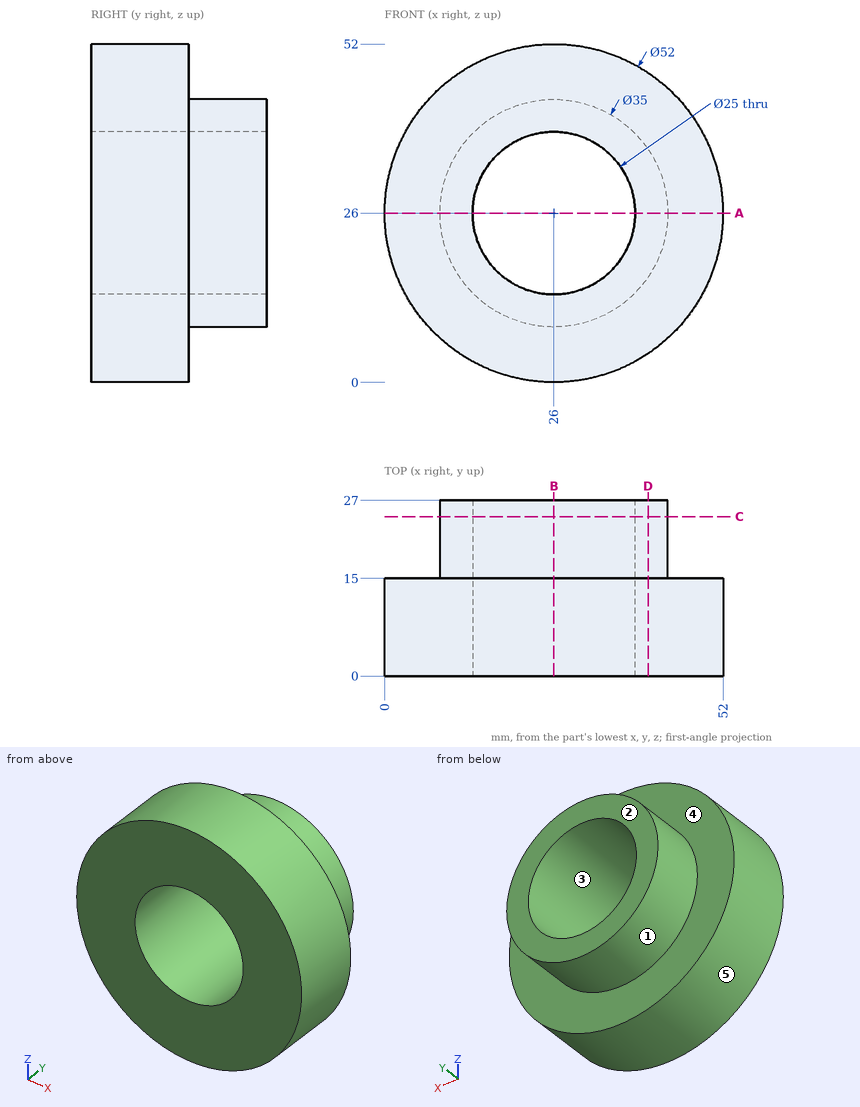
Print and shaded views of the part. All mm, measured from the part's lowest x, y and z. A direction names the side the tool comes from. Coordinates: 2 decimals unless noted, no trailing zeros. Order: outer loops, then holes, each group sorted by start corner. A loop starts at its lowest first (then second) coordinate and runs counter-clockwise, first axis right, second up. Notation, with made-up numbers: (-35, 29.5) - (-7, 29.5) arc R15 ccw to (-7, 47.5) - close; hole circle Ø2 at (48, 64.5). An arc over 180 degrees is marked (long way). Put each result on its own line as item: value.
1. Saw through at D-D (x = 40.5). Write the cut outline in (y, z).
Answer sheet:
outline: (0, 4.42) - (15, 4.42) - (15, 16.2) - (27, 16.2) - (27, 35.8) - (15, 35.8) - (15, 47.58) - (0, 47.58) - close
2. Saw through at C-C (y = 24.5). Write the cut outline in (x, z).
Answer sheet:
outline: circle Ø35 at (26, 26); hole circle Ø25 at (26, 26)
3. Tool access for the marked faces 1 and 2: list every direction of +Z, -Z, +X, -X, +Y, -Y with a clear straight run to the whole face (end or side of a thin tool).
Answer sheet:
face 1: +Y
face 2: +Z, -Z, +X, -X, +Y
4. Drop flat-ended pins along their axis: P1, Ø6, axis at x = 35, y = 16, coming from the +Z side; P2, Ø6, axis at x = 41, y = 5.5, coming from the +Z side; P3, Ø4, axis at y = 10.5, z = 44, coming from the -X side. Give the stop position or say it passes through.
Answer sheet:
P1: stops at z = 51.26
P2: stops at z = 49.07
P3: stops at x = 5.51
5. Probe line 1 along X through (y, z) = (18.25, 26); line 2 along Z through (x, y) = (26, 7.5). List the from-to ranges inside material, lowest first. Write a range as [from, to].
Answer sheet:
line 1: x = [8.5, 13.5], [38.5, 43.5]
line 2: z = [0, 13.5], [38.5, 52]
6. Pull direction X, two halves, no side cores. Call the marked faces 3, 4 and 5: pulls with the +X half, pulls with the -X half, needs draft (parallel to the pull), parting line crosses it, or undercut.
Answer sheet:
face 3: undercut
face 4: needs draft
face 5: parting line crosses it
7. Saw through at B-B (x = 26). Write the cut outline in (y, z), and give its area (3 significant figures).
Answer sheet:
outline: (0, 0) - (15, 0) - (15, 8.5) - (27, 8.5) - (27, 13.5) - (0, 13.5) - close; (0, 38.5) - (27, 38.5) - (27, 43.5) - (15, 43.5) - (15, 52) - (0, 52) - close
area: 525 mm^2
8. Saw through at A-A (z = 26). Write the cut outline in (x, y), and give its area (3 significant figures).
Answer sheet:
outline: (0, 0) - (13.5, 0) - (13.5, 27) - (8.5, 27) - (8.5, 15) - (0, 15) - close; (38.5, 0) - (52, 0) - (52, 15) - (43.5, 15) - (43.5, 27) - (38.5, 27) - close
area: 525 mm^2
